Part model, mm, in its own coordinate system. Face numbers are marked on the shaded views. A direction names the side the tool comes from. Round coordinates to 2 decimals unless told otherwise and drop trailing zeros. Write each loop counter-clockwise with the first axis right and the second up, starting at its lowest first coordinate (ties: lowest second). Pieces come first, ordered by that corner, then holes.
1) Pull direction X, two halves, no side cores. Call the marked faces 1, 2, 3 and 4: +X half, -X half, draft (parallel to the pull), parting line (faces both ways), or undercut.
2) Saw through at C-C on y = 0. Count the separate pieces of the cut face and the enclosed holes in it, and give its area (3 significant figures).
3) Which spindle directions (+Z, -Z, +X, -X, +Y, -Y) get a long thin tool onto all of the face, cutting with end or side? Do the marked faces 5 and 6. Say none if no direction does.
4) Drill centre lines: L1, parallel to X at y = -0.75, z = 4.5; L2, parallel to X at y = -0.5, z = 1.5; L3, parallel to Z at x = -4.25, y = 4. Where is each one in solid material? Low to high.
5) Saw through at A-A on z = 3.5. Write the cut outline in (x, y) (3 decimals), and give its area (3 significant figures).
6) Saw through at B-B on x = 12.25. Write the cut outline in (y, z), and give its area (3 significant figures).
7) Flat gauge pins, fed straight in: pin 1 (11 mm diameter, centred on x = -2.5, y = 2, fed in from +Z); pin 2 (7.5 mm diameter, centred on x = -2.5, y = 2.5, fed in from +Z); pin 3 (1.8 mm diameter, centred on y = -1.5, z = 6, fed in from -X); pin 4 (5 mm diameter, centred on x = -6, z = 2, fed in from +Y). Where does each tip first touch, or does it go through?
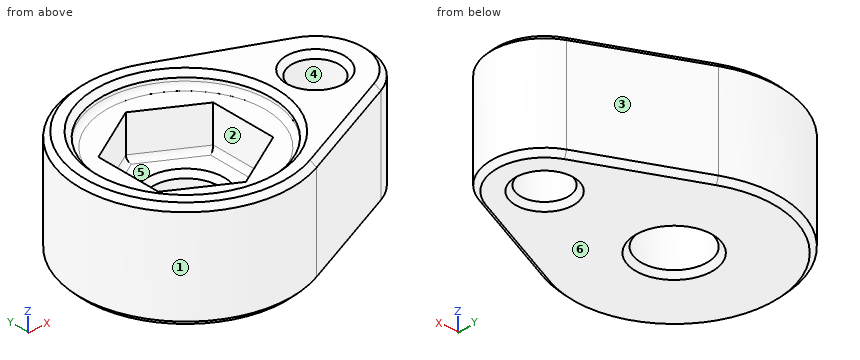
```python
from build123d import *

# Parameters (mm, degrees)
F0_R     = 2.25
F1_DEPTH = 10
F2_R     = 8
F3_DEPTH = 1.3
F5_DEPTH = 4
F6_R     = 3.125
F7_DEPTH = 4.701
F8_R     = 0.5
F9_SIZE  = 0.5


with BuildPart() as f1:
    # F0 (on Top) → F1 (new body)
    with BuildSketch(Plane.XY):
        with BuildLine():
            Line((14.290816, 4.564545), (4.081633, 9.129089))
            ThreePointArc((4.081633, 9.129089), (-10, 0), (4.081633, -9.129089))
            Line((4.081633, -9.129089), (14.290816, -4.564545))
            ThreePointArc((14.290816, -4.564545), (17.25, 0), (14.290816, 4.564545))
        make_face()
        with Locations((12.25, 0)):
            Circle(F0_R, mode=Mode.SUBTRACT)
    extrude(amount=F1_DEPTH)

    # F2 (on face) → F3 (cut)
    with BuildSketch(Plane.XY.offset(10)):
        Circle(F2_R)
    extrude(amount=-F3_DEPTH, mode=Mode.SUBTRACT)

    # F4 (on face) → F5 (cut)
    with BuildSketch(Plane.XY.offset(8.7)):
        Polygon((5.425, -3.132125), (5.425, 3.132125), (0, 6.26425), (-5.425, 3.132125), (-5.425, -3.132125), (0, -6.26425), align=None)
    extrude(amount=-F5_DEPTH, mode=Mode.SUBTRACT)

    # F6 (on face) → F7 (cut, through all)
    with BuildSketch(Plane.XY.offset(4.7)):
        Circle(F6_R)
    extrude(amount=-F7_DEPTH, mode=Mode.SUBTRACT)

    # F8
    f8_edges = [f1.edges().sort_by_distance(p)[0] for p in [
        (-8, 0, 8.7),
        (-2.7125, 4.698188, 4.7),
        (2.7125, 4.698188, 4.7),
        (-5.425, 0, 4.7),
        (-2.7125, -4.698188, 4.7),
        (2.7125, -4.698188, 4.7),
        (5.425, 0, 4.7),
    ]]
    fillet(f8_edges, radius=F8_R)

    # F9
    f9_edges = [f1.edges().sort_by_distance(p)[0] for p in [
        (-8, 0, 10),
        (10, 0, 10),
        (-10, 0, 10),
        (9.186224, -6.846817, 10),
        (-10, 0, 0),
        (9.186224, 6.846817, 0),
        (-3.125, 0, 0),
        (10, 0, 0),
        (-3.125, 0, 4.7),
    ]]
    chamfer(f9_edges, length=F9_SIZE)


solid = f1.part
```
Completed:
1. face 1: parting line
1. face 2: undercut
1. face 3: +X half
1. face 4: undercut
2. separate pieces: 3
2. enclosed holes: 0
2. area: 132 mm2
3. face 5: +Z
3. face 6: -Z, +X, -X, +Y, -Y
4. L1: x = -9.97 to -3.34, 3.34 to 10.13, 14.37 to 17.19
4. L2: x = -9.99 to -3.08, 3.08 to 10.06, 14.44 to 17.22
4. L3: z = 0 to 8.7
5. outline: (4.082, -9.129) - (14.291, -4.565) arc R5 ccw to (14.291, 4.565) - (4.082, 9.129) arc R10 ccw (long way) to start; hole circle Ø6.25 at (0, 0); hole circle Ø4.5 at (12.25, 0)
5. area: 349 mm2
6. outline: (-5.48, 0.5) - (-4.93, 0) - (-2.75, 0) - (-2.25, 0.5) - (-2.25, 9.5) - (-2.75, 10) - (-4.93, 10) - (-5.48, 9.5) - close; (2.25, 0.5) - (2.75, 0) - (4.93, 0) - (5.48, 0.5) - (5.48, 9.5) - (4.93, 10) - (2.75, 10) - (2.25, 9.5) - close
6. area: 63.5 mm2
7. pin 1: stops at z = 10
7. pin 2: stops at z = 8.7
7. pin 3: stops at x = -9.98
7. pin 4: stops at y = 9.37
